Source: CAD feature listing. Evaluate the final solid. Frame: model axes, mm. A direction names the side the tool comes from. Round coordinates to 2 decimals unless told otherwise and drop trailing zeros. Write each loop counter-clockwise with the first axis right and the second up, starting at its lowest first coordinate (ties: lowest second). Pieces come first, ordered by that corner, then holes. Notation, with made-up numbers: (76.25, 2.25) -> (95.25, 2.25) arc R28 ccw to (95.25, 41.25) -> close; hole circle Ø2 at (32.5, 42). An arc over 180 degrees is marked (long way). Put each result on its own line as item: value.
Autodesk Inventor part; units mm, degrees
ref_plane "Work Plane3" through (0, -5.1401, 6.0637) normal (0, 0, 1) x (1, 0, 0)
ref_plane "YZ Plane" through (0, 0, 0) normal (1, 0, 0) x (0, 1, 0)
ref_plane "XZ Plane" through (0, 0, 0) normal (0, 1, 0) x (-1, 0, 0)
sketch "Sketch1" plane through (0, 0, 0) normal (1, 0, 0) x (0, 1, 0)
  line L0 (5.8599, 7.0637) -> (-4.1401, 7.0637)
  line L1 (-4.1401, 7.0637) -> (-4.1401, -2.9363)
  line L2 (-4.1401, -2.9363) -> (5.8599, -2.9363)
  line L3 (5.8599, -2.9363) -> (5.8599, 7.0637)
  line L4 (6.8599, 8.0637) -> (-5.1401, 8.0637)
  line L5 (-5.1401, 8.0637) -> (-5.1401, -3.9363)
  line L6 (-5.1401, -3.9363) -> (6.8599, -3.9363)
  line L7 (6.8599, -3.9363) -> (6.8599, 8.0637)
  point P0 (0, 0)
  dimension "d0" = 10
  dimension "d1" = 10
  dimension "d2" = 12
  dimension "d3" = 12
  dimension "d4" = 1
  dimension "d6" = 1
extrude "Extrusion1" add sketch "Sketch1" along normal blind 100
ref_plane "Work Plane1" through (0, -5.1401, 2.0637) normal (0, 0, 1) x (1, 0, 0)
ref_plane "Work Plane2" through (0, 0.8599, 8.0637) normal (0, 1, 0) x (1, 0, 0)
ref_plane "Work Plane3" through (0, -5.1401, 6.0637) normal (0, 0, 1) x (1, 0, 0)
sketch "Sketch3" plane through (0, -5.1401, 6.0637) normal (0, 0, 1) x (1, 0, 0)
  line L0 (0, 12) -> (100, 12)
  line L1 (10, 12) -> (28, 12)
  line L2 (28, 12) -> (28, 17)
  line L3 (28, 17) -> (10, 17)
  line L4 (10, 17) -> (10, 12)
  line L5 (72, 12) -> (90, 12)
  line L6 (90, 12) -> (90, 17)
  line L7 (90, 17) -> (72, 17)
  line L8 (72, 17) -> (72, 12)
  line L9 (100, 12) -> (100, 0)
  line L10 (0, 12) -> (0, 0)
  line L11 (50, 21.2815) -> (50, -16.5994)
  point P0 (0, 5.1401)
  dimension "d10" = 18
  dimension "d11" = 18
  dimension "d12" = 100
  dimension "d13" = 50
  dimension "d15" = 10
  dimension "d16" = 10
  dimension "d17" = 5
extrude "Extrusion2" add sketch "Sketch3" along normal blind 1
mirror "Mirror1" about plane through (0, -5.1401, 2.0637) normal (0, 0, 1) of "Extrusion2"
mirror "Mirror2" about plane through (0, 0.8599, 8.0637) normal (0, 1, 0) of "Extrusion2", "Mirror1"
pattern_circular "Circular Pattern1" count 2 over 270 about axis through (0, 0.8599, 2.0637) along (-1, 0, 0) of "Extrusion2", "Mirror1"
equation "\"d1\" = d0"
equation "\"d3\" = d2"
equation "\"d11\" = d10"
equation "\"d13\" = 0.5 * d12"
equation "\"d15\" = 0.1 * d12"
equation "\"d16\" = d15"
properties part number "fuselage_tail_interface"
Q1. Pin query (flat end, axial travel): pin 1 (0.8 mm diameter, centred on y = 9.5, z = 6.5, fed in from +X); pin 2 (1 mm diameter, centred on x = 79, y = -5.5, fed in from -Z); pin 3 (0.5 mm diameter, centred on y = -7, z = -2, fed in from -X); pin 4 (2.5 mm diameter, centred on x = 82.5, z = 9.5, fed in from +Y). Return the tip coordinate at first contact, or that it passes through.
Ans:
pin 1: stops at x = 90
pin 2: stops at z = -3.94
pin 3: stops at x = 10
pin 4: stops at y = 5.86
Q2. Cut plane D-D on z = 9. Output: boundary loops of the cut face in (x, y), and give its area (3 significant figures).
Ans:
outline: (10, -4.14) -> (28, -4.14) -> (28, -3.14) -> (10, -3.14) -> close; (10, 4.86) -> (28, 4.86) -> (28, 5.86) -> (10, 5.86) -> close; (72, -4.14) -> (90, -4.14) -> (90, -3.14) -> (72, -3.14) -> close; (72, 4.86) -> (90, 4.86) -> (90, 5.86) -> (72, 5.86) -> close
area: 72.0 mm^2
Q3. Cut plane B-B on z = -1. Output: boundary loops of the cut face in (x, y), and give its area (3 significant figures).
Ans:
outline: (0, -5.14) -> (100, -5.14) -> (100, -4.14) -> (0, -4.14) -> close; (0, 5.86) -> (100, 5.86) -> (100, 6.86) -> (0, 6.86) -> close
area: 200 mm^2
Q4. Reachability of faces 5 (the flat face through (81, -8, -1.936)), 6 (the flat face through (19, 9, 6.064)), 7 (the flat face through (19, -3.14, 11)), 8 (the flat face through (19, 5.86, 11)) from +Z, -Z, +X, -X, +Y, -Y: full face, straight path, thin tool, end or side. Return the list, or none.
Ans:
face 5: +X, -X, -Y
face 6: +X, -X, +Y
face 7: +Z, +X, -X
face 8: +Z, +X, -X, +Y
Q5. Cut plane A-A on y = 1. Output: boundary loops of the cut face in (x, z).
Ans:
outline: (0, -3.94) -> (100, -3.94) -> (100, -2.94) -> (0, -2.94) -> close; (0, 7.06) -> (100, 7.06) -> (100, 8.06) -> (0, 8.06) -> close
Q6. Material intervals for line 1 (Z direction, x = 67.5, y = 2); line 2 (Z direction, x = 74.5, y = 7.25); line 3 (Y direction, x = 10.5, z = 9.75), sorted ascending. Write a range as [from, to].
Ans:
line 1: z = [-3.94, -2.94], [7.06, 8.06]
line 2: z = [-2.94, -1.94], [6.06, 7.06]
line 3: y = [-4.14, -3.14], [4.86, 5.86]
Q7. Cut plane C-C on x = 61.5. Output: boundary loops of the cut face in (y, z), and give its area (3 significant figures).
Ans:
outline: (-5.14, -3.94) -> (6.86, -3.94) -> (6.86, 8.06) -> (-5.14, 8.06) -> close; hole (-4.14, -2.94) -> (5.86, -2.94) -> (5.86, 7.06) -> (-4.14, 7.06) -> close
area: 44.0 mm^2
Q8. Draft query along Z for faces 1 (the flat face through (19, -8, -2.936)), 2 (the flat face through (81, -4.14, 11)), 3 (the flat face through (81, -8, 6.064)), 4 (the flat face through (81, 9, 7.064)). Return one class per face: +Z half, -Z half, draft (parallel to the pull), parting line (faces both ways), or undercut.
Ans:
face 1: -Z half
face 2: draft
face 3: undercut
face 4: +Z half
